```python
from build123d import *

# Parameters (mm, degrees)
F1_DEPTH = 32
F3_DEPTH = 25
F4_DEPTH = 40
F5_DEPTH = 32
F0_W     = 16
F0_H     = 8
F6_DEPTH = 25
F7_DEPTH = 13
F8_DEPTH = 5


with BuildPart() as f1:
    # F0 (on Top) → F1 (new body)
    with BuildSketch(Plane.XY):
        Polygon((12, -20), (20, -20), (20, 12), (12, 12), (12, 4), (12, -4), (12, -12), align=None)
    extrude(amount=F1_DEPTH)

    # F2 (on face) → F3 (cut)
    with BuildSketch(Plane.YZ.offset(20)):
        Polygon((-20, 0), (12, 32), (-20, 32), align=None)
    extrude(amount=-F3_DEPTH, mode=Mode.SUBTRACT)

    # F0 (on Top) → F4 (join)
    with BuildSketch(Plane.XY):
        Polygon((12, 12), (20, 12), (20, 20), (-12, 20), (-20, 20), (-20, -20), (-12, -20), (-12, 12), align=None)
    extrude(amount=F4_DEPTH)

    # F0 (on Top) → F5 (join)
    with BuildSketch(Plane.XY):
        Polygon((-12, -20), (-4, -20), (-4, -12), (-4, -4), (-4, 4), (12, 4), (12, 12), (-12, 12), align=None)
    extrude(amount=F5_DEPTH)

    # F0 (on Top) → F6 (join)
    with BuildSketch(Plane.XY):
        with Locations((4, 0)):
            Rectangle(F0_W, F0_H)
    extrude(amount=F6_DEPTH)

    # F0 (on Top) → F7 (join)
    with BuildSketch(Plane.XY):
        with Locations((4, -8)):
            Rectangle(F0_W, F0_H)
    extrude(amount=F7_DEPTH)

    # F0 (on Top) → F8 (join)
    with BuildSketch(Plane.XY):
        with Locations((4, -16)):
            Rectangle(F0_W, F0_H)
    extrude(amount=F8_DEPTH)


solid = f1.part
```
Build history of the part. All positions in model axes, mm. A direction names the side the tool comes from. Round coordinates to 2 decimals unless told otherwise and drop trailing zeros. Loops run counter-clockwise (first coordinate to the right, second up) from the corner with the lowest first, then second, coordinate; pieces in that order, holes last. Notation, with made-up numbers: M 58,74.5 L 69,74.5 A29 cw 69,98.5 Z; hole C 82.5,79 d11. An arc over 180 degrees is marked long. Answer as CSV lines item,"result".
1. Cut at D-D on y = 1.5. Write the cut outline in (x, z), then the cut area to 3 significant figures.
Resolved:
outline,"M -20,0 L 20,0 L 20,21.5 L 12,21.5 L 12,25 L -4,25 L -4,32 L -12,32 L -12,40 L -20,40 Z"
area,"1,150 mm²"
2. Flat gauge pins, fed straight in: P1, Ø6.5, axis at x = 0.5, y = -9.5, coming from the +Z side; P2, Ø6.5, axis at y = -0.5, z = 36.5, coming from the +X side; P3, Ø2.5, axis at x = 5.5, y = -17, coming from the +Z side. Where does each tip first touch, or does it go through?
Resolved:
P1,"stops at z = 13"
P2,"stops at x = -12"
P3,"stops at z = 5"
3. Wall check: probe 1 along Z at (x, y) = (-11, 6.5); probe 2 along Z at (x, y) = (10.5, 1); probe 3 along X at (y, z) = (-13, 12). Give the ranges that are in metal, low to high. Write a range as [from, to].
Resolved:
probe 1,"z = [0, 32]"
probe 2,"z = [0, 25]"
probe 3,"x = [-20, -4]"
4. Cut at B-B on x = 9.5. Write the cut outline in (y, z), then the cut area to 3 significant figures.
Resolved:
outline,"M -20,0 L 20,0 L 20,40 L 12,40 L 12,32 L 4,32 L 4,25 L -4,25 L -4,13 L -12,13 L -12,5 L -20,5 Z"
area,"920 mm²"
5. 3-axis set-ups, long thin cutter, end or side, ignore diameter. For faces 1 (the flat face through (-20, 0, 20)), 2 (the flat face through (4, 0, 25)), 3 (the flat face through (4, -16, 5)): which of +Z, -Z, +X, -X, +Y, -Y reach the whole face in a straight line?
Resolved:
face 1,"+Z, -Z, -X, +Y, -Y"
face 2,"+Z, +X, -Y"
face 3,"+Z, -Y"
6. Cut at C-C on y = 6.5. Write the cut outline in (x, z), then the cut area to 3 significant figures.
Resolved:
outline,"M -20,0 L 20,0 L 20,26.5 L 12,26.5 L 12,32 L -12,32 L -12,40 L -20,40 Z"
area,"1,300 mm²"
7. Two-plate mould, pull along X, no slides. Class faces 4 (the flat face through (4, -12, 9)), 5 (the flat face through (-6, 0, 32)), 6 (the flat face through (20, 9, 15)): released by +X, released by -X, zero draft, split by the parting line, or undercut.
Resolved:
face 4,"undercut"
face 5,"zero draft"
face 6,"released by +X"
8. Cut at A-A on z = 23.5. Write the cut outline in (x, y), then the cut area to 3 significant figures.
Resolved:
outline,"M -20,-20 L -4,-20 L -4,-4 L 12,-4 L 12,3.5 L 20,3.5 L 20,20 L -20,20 Z"
area,"1,160 mm²"
